from build123d import *

# Parameters (mm, degrees)
SKETCH1_R           = 7
BOSS_EXTRUDE1_DEPTH = 60
SKETCH1_3_R         = 7
BOSS_EXTRUDE2_DEPTH = 66


with BuildPart() as part:
    # Sketch1 → Boss-Extrude1 (new body)
    with BuildSketch(Plane(origin=(0, 0, 0), x_dir=(1, 0, 0), z_dir=(0, 1, 0))):
        Polygon((12.124355653, 0), (6.062177826, 10.5), (-6.062177826, 10.5), (-12.124355653, 0), (-6.062177826, -10.5), (6.062177826, -10.5), align=None)
        with Locations(Location((0, 0, 0), (0, 0, 270))):
            Circle(SKETCH1_R, mode=Mode.SUBTRACT)
    extrude(amount=BOSS_EXTRUDE1_DEPTH)

    # Sketch1_3 → Boss-Extrude2 (add)
    with BuildSketch(Plane(origin=(0, 0, 0), x_dir=(1, 0, 0), z_dir=(0, 1, 0))):
        with Locations(Location((0, 0, 0), (0, 0, 270))):
            Circle(SKETCH1_3_R)
    extrude(amount=BOSS_EXTRUDE2_DEPTH)


solid = part.part
CAD build for the part. Positions are in the model's coordinates, mm. A direction names the side the tool comes from. Coordinates: 2 decimals unless noted, no trailing zeros. Loops run counter-clockwise (first coordinate to the right, second up) from the corner with the lowest first, then second, coordinate; pieces in that order, holes last. Notation, with made-up numbers: (82, 76.5) -> (119, 76.5) arc R14 cw to (119, 85.5) -> close; hole circle Ø4 at (36, 68). An arc over 180 degrees is marked (long way). One line per item, written item: value.
1. Which spindle directions (+Z, -Z, +X, -X, +Y, -Y) get a long thin tool onto all of the face, cutting with end or side? Do faces 1 (the face through (-6.834, 62.958, -1.517)), 2 (the face through (9.051, 29.58, 5.324)). Say none if no direction does.
Answers:
face 1: +Y
face 2: +Z, +X, +Y, -Y
2. Slice it at A-A on x = 0. Write the cut outline in (y, z).
Answers:
outline: (0, -10.5) -> (60, -10.5) -> (60, -7) -> (66, -7) -> (66, 7) -> (60, 7) -> (60, 10.5) -> (0, 10.5) -> close
3. Slice it at B-B on z = -1. Write the cut outline in (x, y).
Answers:
outline: (-11.55, 0) -> (11.55, 0) -> (11.55, 60) -> (6.93, 60) -> (6.93, 66) -> (-6.93, 66) -> (-6.93, 60) -> (-11.55, 60) -> close
4. Flat gauge pins, fed straight in: P1, Ø6, axis at x = -9.5, y = 52.5, coming from the -Z side; P2, Ø8, axis at x = -7.5, z = -8, coming from the -Y side; P3, Ø6, axis at y = 25.5, z = -1, coming from the -X side; P4, Ø12, axis at y = 11, z = -6.5, coming from the +X side. Where does each tip first touch, or does it go through?
Answers:
P1: stops at z = -9.74
P2: stops at y = 0
P3: stops at x = -12.12
P4: stops at x = 11.84
5. Slice it at D-D on z = -8.75. Write the cut outline in (x, y), and give its area (3 significant figures).
Answers:
outline: (-7.07, 0) -> (7.07, 0) -> (7.07, 60) -> (-7.07, 60) -> close
area: 849 mm^2
6. Drill centre lines: line 1 (Y direction, x = 5.75, z = 7.25); line 2 (X direction, y = 18, z = -7.75); line 3 (X direction, y = 30, z = -6.5). Where is each one in solid material? Low to high. Write a range as [from, to].
Answers:
line 1: y = [0, 60]
line 2: x = [-7.65, 7.65]
line 3: x = [-8.37, 8.37]
7. Slice it at C-C on y = 8.5. Write the cut outline in (x, z).
Answers:
outline: (-12.12, 0) -> (-6.06, -10.5) -> (6.06, -10.5) -> (12.12, 0) -> (6.06, 10.5) -> (-6.06, 10.5) -> close
